Geometry check sheet. Reference: the model listing, model coordinates, mm. Give positions to 0.01 mm unless a question says otherwise; leave off trailing zeros. Answer as a JSON object with one key per item and string values.
from build123d import *

# Parameters (mm, degrees)
SKETCH_R  = 2.25
PAD_DEPTH = 400
FILLET_R  = 1.5


with BuildPart() as part:
    # Sketch → Pad (new body)
    with BuildSketch(Plane(origin=(0, 0, 0), x_dir=(1, 0, 0), z_dir=(0, 0, -1))):
        Polygon((7, 0), (7, -1), (4, -1), (4, -2.5), (6.499998, -5), (13.500002, -5), (16, -2.5), (16, -1), (13, -1), (13, 0), (20, 0), (20, -7), (19, -7), (19, -4), (17.5, -4), (15.000002, -6.5), (15.000002, -13.500005), (17.5, -16.000005), (19, -16.000005), (19, -13.000005), (20, -13.000005), (20, -20.000005), (13, -20.000005), (7, -20.000005), (0, -20.000005), (0, -13.000005), (0, -7), (0, 0), align=None)
        with Locations((10, -10.000002)):
            Circle(SKETCH_R, mode=Mode.SUBTRACT)
        Polygon((7, -19.000005), (4, -19.000005), (4, -17.500005), (6.499998, -15.000005), (13.500002, -15.000005), (16, -17.500005), (16, -19.000005), (13, -19.000005), align=None, mode=Mode.SUBTRACT)
        Polygon((1, -7), (1, -4), (2.5, -4), (4.999998, -6.5), (4.999998, -13.500005), (2.5, -16.000005), (1, -16.000005), (1, -13.000005), align=None, mode=Mode.SUBTRACT)
    extrude(amount=PAD_DEPTH)

    # Fillet
    fillet_edges = [part.edges().sort_by_distance(p)[0] for p in [
        (0, 20.000005, -200),
        (0, 0, -200),
        (20, 0, -200),
        (20, 20.000005, -200),
    ]]
    fillet(fillet_edges, radius=FILLET_R)


solid = part.part
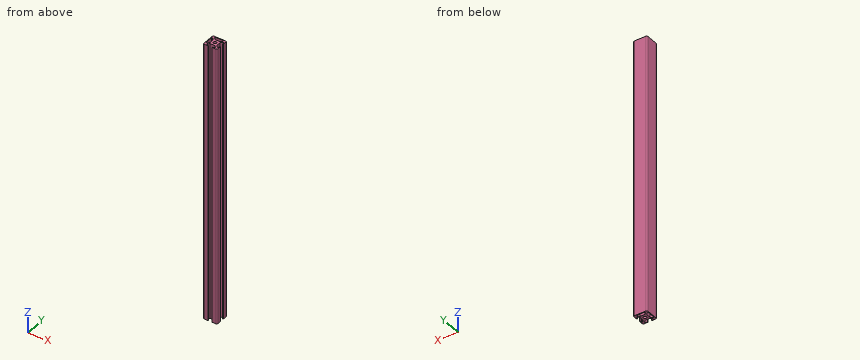
1) Material ranges on line 1 along Y through (x, z) = (10, -95.5); line 2 along Y through (x, z) = (5.5, -279); line 3 along X through (y, z) = (3.5, -259.5), recorded low to high. Write a range as from..to.
Geometry check:
{"line 1": "y = 5..7.75, 12.25..15, 19..20", "line 2": "y = 0..1, 4..16, 19..20", "line 3": "x = 0..5, 15..20"}
2) Depth check by flat-ended pin: P1, Ø7, axis at x = 10, y = 10, coming from the -Z side; P2, Ø3.5, axis at y = 10, z = -262.5, coming from the +X side; P3, Ø0.8, axis at y = 0.5, z = -181, coming from the +X side; P4, Ø1.5, axis at x = 10, z = -227.5, coming from the -Y side. Enter the tip coordinate at first touch or a pass-through.
Geometry check:
{"P1": "stops at z = -400", "P2": "stops at x = 15", "P3": "stops at x = 19.87", "P4": "stops at y = 5"}
3) Section check A-A on z = -179.5. Count the separate pieces of the cut face and the enclosed holes in it, plus the area to 3 significant figures.
Geometry check:
{"separate pieces": "1", "enclosed holes": "3", "area": "203 mm2"}
